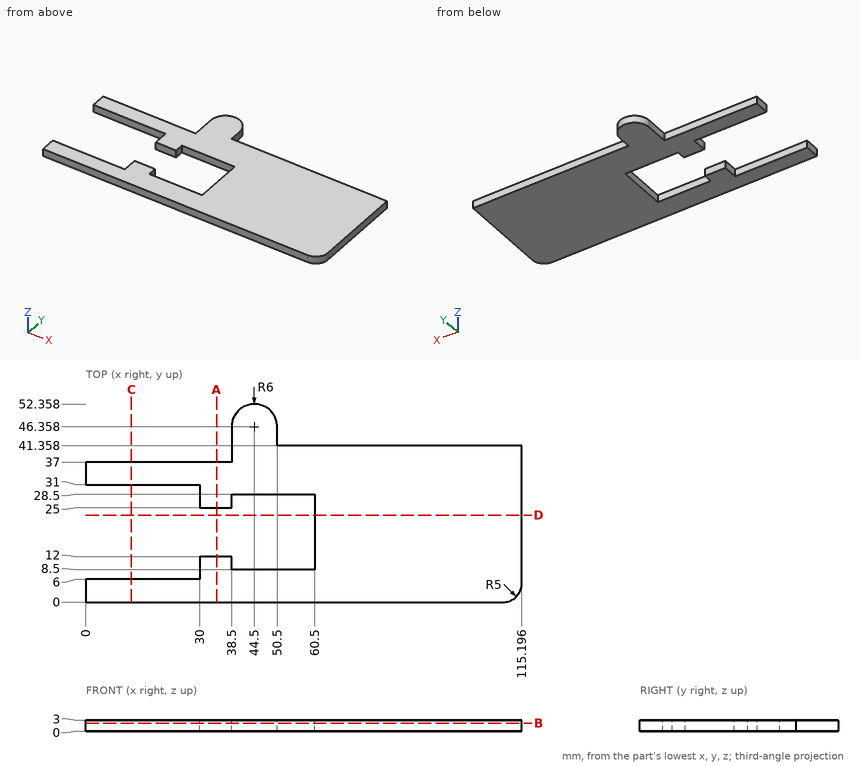
Geometry check sheet. Reference: drawing and pictorial views, mm from the part's lowest x, y, z. Coordinates: 2 decimals unless noted, no trailing zeros. Loops run counter-clockwise (first coordinate to the right, second up) from the corner with the lowest first, then second, coordinate; pieces in that order, holes last. Notation, with made-up numbers: (-28.5, -38.75) -> (-1.5, -38.75) arc R23 cw to (-1.5, -9.75) -> close; hole circle Ø8 at (-13.5, -25.75). An arc over 180 degrees is marked (long way). Put each result on its own line as item: value.
1) Thickness scan on line 1 (Y direction, x = 31.5, z = 2.2); line 2 (Y direction, x = 6.5, z = 0.3); line 3 (X direction, y = 26, z = 1.7). Record the ranges inside material, lowest first.
Result set:
line 1: y = 0 to 12, 25 to 37
line 2: y = 0 to 6, 31 to 37
line 3: x = 30 to 38.5, 60.5 to 115.2
2) Cross-section at C-C on x = 12. Record the boundary of the cut face in (y, z).
Result set:
outline: (0, 0) -> (6, 0) -> (6, 3) -> (0, 3) -> close; (31, 0) -> (37, 0) -> (37, 3) -> (31, 3) -> close
3) Cross-section at B-B on z = 2.2. Record the boundary of the cut face in (x, y).
Result set:
outline: (0, 0) -> (110.2, 0) arc R5 ccw to (115.2, 5) -> (115.2, 41.36) -> (50.5, 41.36) -> (50.5, 46.36) arc R6 ccw to (38.5, 46.36) -> (38.5, 37) -> (0, 37) -> (0, 31) -> (30, 31) -> (30, 25) -> (38.5, 25) -> (38.5, 28.5) -> (60.5, 28.5) -> (60.5, 8.5) -> (38.5, 8.5) -> (38.5, 12) -> (30, 12) -> (30, 6) -> (0, 6) -> close
4) Gauge pin test, flat ends, axial feed: pin 1 Ø0.9 at (x, z) = (10.5, 2) entering from +Y; pin 2 Ø1.5 at (y, z) = (7.5, 1.5) entering from -X. Record the tip position at first contact, or that the pin passes through.
Result set:
pin 1: stops at y = 37
pin 2: stops at x = 30
5) Cross-section at A-A on x = 34.5. Record the boundary of the cut face in (y, z).
Result set:
outline: (0, 0) -> (12, 0) -> (12, 3) -> (0, 3) -> close; (25, 0) -> (37, 0) -> (37, 3) -> (25, 3) -> close
6) Cross-section at D-D on y = 23. Record the boundary of the cut face in (x, z).
Result set:
outline: (60.5, 0) -> (115.2, 0) -> (115.2, 3) -> (60.5, 3) -> close
